from build123d import *

# Parameters (mm, degrees)
SKETCH011_W                                = 24
SKETCH011_H                                = 18
SKETCH011_R                                = 4
PAD001007004004002003004004002012002_DEPTH = 30
CHAMFER_SIZE                               = 6
SKETCH012_W                                = 50
SKETCH012_H                                = 30
PAD001007004004002003004004002012003_DEPTH = 5
CHAMFER001_SIZE                            = 4


with BuildPart() as part:
    # Sketch011 → Pad001007004004002003004004002012002 (new body)
    with BuildSketch(Plane.XZ):
        Rectangle(SKETCH011_W, SKETCH011_H)
        Circle(SKETCH011_R, mode=Mode.SUBTRACT)
    extrude(amount=PAD001007004004002003004004002012002_DEPTH)

    # Chamfer
    chamfer_edges = [part.edges().sort_by_distance(p)[0] for p in [
        (12, -15, 9),
        (-12, -15, 9),
    ]]
    chamfer(chamfer_edges, length=CHAMFER_SIZE)

    # Sketch012 → Pad001007004004002003004004002012003 (new body)
    with BuildSketch(Plane(origin=(0, 0, -9), x_dir=(1, 0, 0), z_dir=(0, 0, -1))):
        with Locations((0, 15)):
            Rectangle(SKETCH012_W, SKETCH012_H)
    extrude(amount=-PAD001007004004002003004004002012003_DEPTH)

    # Chamfer001
    chamfer001_edges = [part.edges().sort_by_distance(p)[0] for p in [
        (12, -15, -4),
        (-12, -15, -4),
        (-25, -15, -4),
        (25, -15, -4),
    ]]
    chamfer(chamfer001_edges, length=CHAMFER001_SIZE)


solid = part.part
The model under review builds one solid part; all positions refer to its coordinate system, in mm. A direction names the side the tool comes from. Round coordinates to 2 decimals unless told otherwise and drop trailing zeros. Loops run counter-clockwise (first coordinate to the right, second up) from the corner with the lowest first, then second, coordinate; pieces in that order, holes last. Notation, with made-up numbers: (53.5, 11.25) -> (110.5, 11.25) arc R17 cw to (110.5, 16.25) -> close; hole circle Ø10 at (58, 10). An arc over 180 degrees is marked (long way). Answer as CSV lines item,"result".
1) Tool access review of faces 1 (the face through (12, -15, 1)), 2 (the face through (-12, -15, 1)), 3 (the face through (0, -15, 9)): name each direction out of +Z, -Z, +X, -X, +Y, -Y from which nothing blocks a thin tool from reaching the whole face with its end or side.
Geometry results:
face 1,"+Z, +X, +Y, -Y"
face 2,"+Z, -X, +Y, -Y"
face 3,"+Z, +X, -X, +Y, -Y"
2) Draft analysis for pull direction Z (two halves, no side actions). For faces 4 (the face through (9, -15, 6)), 5 (the face through (-0.867, -14.79, -3.905)), 6 (the face through (0, -15, -9)), 7 (the face through (-25, -14.8, -8.5)), state which applies: pulls with the +Z half, pulls with the -Z half, needs draft (parallel to the pull), parting line crosses it, or undercut.
Geometry results:
face 4,"pulls with the +Z half"
face 5,"undercut"
face 6,"pulls with the -Z half"
face 7,"needs draft"
3) Add section A-A on x = 0. Write out the cut boundary in (y, z), plus the area to 3 significant figures.
Geometry results:
outline,"(-30, -9) -> (0, -9) -> (0, -4) -> (-30, -4) -> close; (-30, 4) -> (0, 4) -> (0, 9) -> (-30, 9) -> close"
area,"300 mm²"
4) Add section D-D on x = -13. Write out the cut boundary in (y, z), plus the area to 3 significant figures.
Geometry results:
outline,"(-30, -9) -> (0, -9) -> (0, -1) -> (-30, -1) -> close"
area,"240 mm²"
5) For P1, Ø9, axis at x = 0, z = 0, coming from the -Y side; P2, Ø2.5, axis at x = 18, y = -21.5, coming from the +Z side; P3, Ø0.9, axis at y = -19.5, z = 1, coming from the +X side; P4, Ø10, axis at x = -18, y = -4.5, coming from the +Z side, all flat-tipped, find the tip position at first contact; note any pin that passes through.
Geometry results:
P1,"stops at y = -30"
P2,"stops at z = -4"
P3,"stops at x = 12"
P4,"stops at z = -1"
6) To check wall thickness, follow line 1 along Z through (x, y) = (0, -27); line 2 along Z through (x, y) = (-21, -26); line 3 along X through (y, z) = (-11.25, 0). State the ranges of each line that lie inside material, in increasing order. Write a range as from..to.
Geometry results:
line 1,"z = -9..-4, 4..9"
line 2,"z = -9..-4"
line 3,"x = -12..-4, 4..12"
7) Add section B-B on y = -11. Write out the cut boundary in (x, z).
Geometry results:
outline,"(-25, -9) -> (25, -9) -> (25, -8) -> (21, -4) -> (16, -4) -> (12, 0) -> (12, 3) -> (6, 9) -> (-6, 9) -> (-12, 3) -> (-12, 0) -> (-16, -4) -> (-21, -4) -> (-25, -8) -> close; hole circle Ø8 at (0, 0)"
8) Add section C-C on z = -2. Write out the cut boundary in (x, y).
Geometry results:
outline,"(-14, -30) -> (-3.46, -30) -> (-3.46, 0) -> (-14, 0) -> close; (3.46, -30) -> (14, -30) -> (14, 0) -> (3.46, 0) -> close"
